```python
from build123d import *

# Parameters (mm, degrees)
BOSS_EXTRUDE1_DEPTH = 6
SKETCH2_R           = 1.5
CUT_EXTRUDE1_DEPTH  = 6


with BuildPart() as part:
    # Sketch1 → Boss-Extrude1 (new body)
    with BuildSketch(Plane(origin=(0, 0, 0), x_dir=(0, 0, -1), z_dir=(1, 0, 0))):
        Polygon((0, 0), (-20, 0), (-20, 1.5), (-11, 1.5), (-11, 4.5), (-20, 4.5), (-20, 6), (-9, 6), (-9, 4.5), (0, 4.5), (0, 3), (-9, 3), (-9, 1.5), (0, 1.5), align=None)
    extrude(amount=BOSS_EXTRUDE1_DEPTH)

    # Sketch2 → Cut-Extrude1 (cut)
    with BuildSketch(Plane.XZ):
        with Locations((3, 3)):
            Circle(SKETCH2_R)
        with Locations((3, 17)):
            Circle(SKETCH2_R)
    extrude(amount=-CUT_EXTRUDE1_DEPTH, mode=Mode.SUBTRACT)


solid = part.part
```
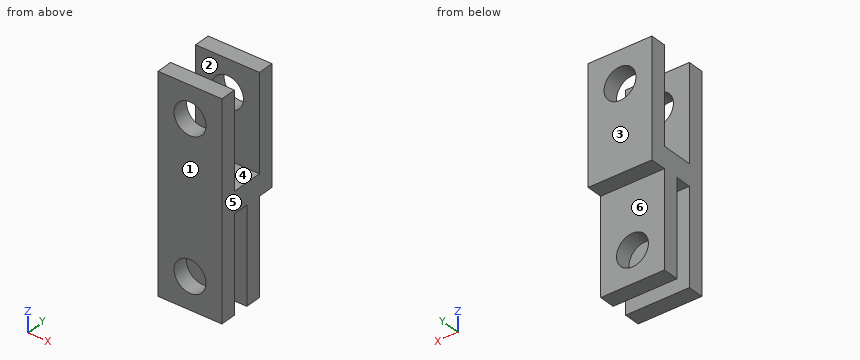
The listing builds one solid part. Answer for the finished solid, in the listing's coordinates (mm). Face numbers are marked on the shaded views. A direction names the side the tool comes from. Round coordinates to 2 decimals unless told otherwise and drop trailing zeros. Loops run counter-clockwise (first coordinate to the right, second up) from the corner with the lowest first, then second, coordinate; pieces in that order, holes last. Notation, with made-up numbers: (57, 32) - (91, 32) arc R21 cw to (91, 47) - close; hole circle Ø9 at (52.5, 9.25). An arc over 180 degrees is marked (long way). Return JSON: item names as keys, results as strings. Group by question number.
1. The part is cut by section A-A on z = 3. Determine the outline of the cut face in (x, y).
2. The part is cut by section B-B on x = 3. State how many separate pieces and enclosed holes the cut face has, then the cut area to 3 significant figures.
3. The part is cut by section C-C on z = 14.5. Determine the outline of the cut face in (x, y).
4. The part is cut by section D-D on y = 3.65. Determine the outline of the cut face in (x, z), then the cut area to 3 significant figures.
5. The mould has two halves that part along Y. Classify the marked faces 1, 2 and 3: pulls with the +Y half, pulls with the -Y half, needs draft (parallel to the pull), parting line crosses it, or undercut.
6. Which of the six approach directions +Z, -Z, +X, -X, +Y, -Y give full straight-line access (tool end or side, diameter ignored) to the marked faces 4, 5 and 6?
7. Each of these flat-tipped pins is pushed along its axis until it touches: P1, Ø1.8, axis at x = 2, z = 6, coming from the +Y side; P2, Ø0.9, axis at x = 3.5, y = 3, coming from the +Z side; P3, Ø1, axis at x = 1, y = 5.5, coming from the -Z side. Where does it stop, or does it pass through?
8. Consider probe 1 along Z at (x, y) = (3, 0.3); probe 2 along Y at (x, z) = (1.1, 2); probe 3 along Y at (x, z) = (2.55, 15). Determine where each line is inside the solid, lowest interval first.
Resolved:
{
 "1": {"outline": "(0, 0) - (1.5, 0) - (1.5, 1.5) - (0, 1.5) - close; (0, 3) - (1.5, 3) - (1.5, 4.5) - (0, 4.5) - close; (4.5, 0) - (6, 0) - (6, 1.5) - (4.5, 1.5) - close; (4.5, 3) - (6, 3) - (6, 4.5) - (4.5, 4.5) - close"},
 "2": {"separate pieces": "5", "enclosed holes": "0", "area": "48.0 mm²"},
 "3": {"outline": "(0, 0) - (6, 0) - (6, 1.5) - (0, 1.5) - close; (0, 4.5) - (6, 4.5) - (6, 6) - (0, 6) - close"},
 "4": {"outline": "(0, 0) - (6, 0) - (6, 11) - (0, 11) - close; hole circle Ø3 at (3, 3)", "area": "58.9 mm²"},
 "5": {"face 1": "pulls with the -Y half", "face 2": "undercut", "face 3": "pulls with the +Y half"},
 "6": {"face 4": "+Z, +X, -X", "face 5": "+Z, -Z, +X, +Y, -Y", "face 6": "-Z, +X, -X, +Y"},
 "7": {"P1": "stops at y = 4.5", "P2": "stops at z = 11", "P3": "stops at z = 9"},
 "8": {"probe 1": "z = 0 to 1.5, 4.5 to 15.5, 18.5 to 20", "probe 2": "y = 0 to 1.5, 3 to 4.5", "probe 3": "y = 0 to 1.5, 4.5 to 6"}
}
